Verification items for the finished model (mm, model axes). Coordinates: 2 decimals unless noted, no trailing zeros. Order: outer loops, then holes, each group sorted by start corner. A loop starts at its lowest first (then second) coordinate and runs counter-clockwise, first axis right, second up. Notation, with made-up numbers: (66, 20.5) - (89, 20.5) arc R14 ccw to (89, 37.5) - close; hole circle Ø3 at (73, 14.25). An arc over 180 degrees is marked (long way). Answer as CSV lines item,"result". Start each with the question number.
1. Section check A-A (y = 0). Record the cut outline in (x, z).
2. Section check C-C (x = 1.25). Record the cut outline in (y, z).
3. Go/stop test with flat-tipped pins: pin 1 (8 mm diameter, centred on y = -6, z = -0.5, fed in from +X); pin 2 (2 mm diameter, centred on x = 7.5, y = 5, fed in from -Z). Record where each tip stops, or that it passes through.
4. Material ranges on L1, parallel to Z at x = 7.75, y = 5.25; L2, parallel to Y at x = 7.5, z = -5.5; L3, parallel to X at y = -6.5, z = 1.5, recorded low to high. Write a range as [from, to].
5. Section check D-D (x = 3.25). Record the cut outline in (y, z), and give its area (3 significant figures).
from build123d import *

# Parameters (mm, degrees)
SKETCH_1_R       = 8
EXTRUDE_1_DEPTH  = 9
CHAMFER_1_SIZE   = 0.357142857
CHAMFER_1_SIZE_2 = 0.5
CHAMFER_2_SIZE   = 0.5


with BuildPart() as part:
    # Эскиз1 → Бобышка-Вытянуть1 (new body)
    with BuildSketch(Plane(origin=(0, 0, 0), x_dir=(0, 0, -1), z_dir=(1, 0, 0))):
        Circle(SKETCH_1_R)
    extrude(amount=EXTRUDE_1_DEPTH)

    # Эскиз2 → Вырез-Повернуть1 (revolve, cut)
    with BuildSketch(Plane.XY):
        with BuildLine():
            Line((-3, 0), (12, 0))
            ThreePointArc((12, 0), (4.5, 7.5), (-3, 0))
        make_face()
    revolve(axis=Axis((0, 0, 0), (1, 0, 0)), mode=Mode.SUBTRACT)

    # Фаска1
    # the kernel refuses this chamfer: 0.5, 0.357142857 mm, written as the material it takes off along each edge
    with BuildSketch(Plane(origin=(9, 0, 0), x_dir=(0, 1, 0), z_dir=(0, 0, 1))) as chamfer_1_piece_1:
        with BuildLine():
            Line((6 + CHAMFER_1_SIZE, 0), (6.296419414, 0.425064103))
            ThreePointArc((6.296419414, 0.425064103), (6.1560674, 0.215979206), (6, 0))
            Line((6, 0), (6 + CHAMFER_1_SIZE, 0))
        make_face()
    revolve(axis=Axis((9, 0, 0), (-1, 0, 0)), mode=Mode.SUBTRACT)
    with BuildSketch(Plane(origin=(0, 0, 0), x_dir=(0, 1, 0), z_dir=(0, 0, 1))) as chamfer_1_piece_2:
        with BuildLine():
            Line((6 + CHAMFER_1_SIZE_2, 0), (6.208166664, -0.291833336))
            ThreePointArc((6.208166664, -0.291833336), (6.10678692, -0.146018659), (6, 0))
            Line((6, 0), (6 + CHAMFER_1_SIZE_2, 0))
        make_face()
    revolve(axis=Axis((0, 0, 0), (-1, 0, 0)), mode=Mode.SUBTRACT)

    # Фаска2
    chamfer_2_edges = [part.edges().sort_by_distance(p)[0] for p in [
        (0, 0, 8),
        (9, 0, 8),
    ]]
    chamfer(chamfer_2_edges, length=CHAMFER_2_SIZE)


solid = part.part
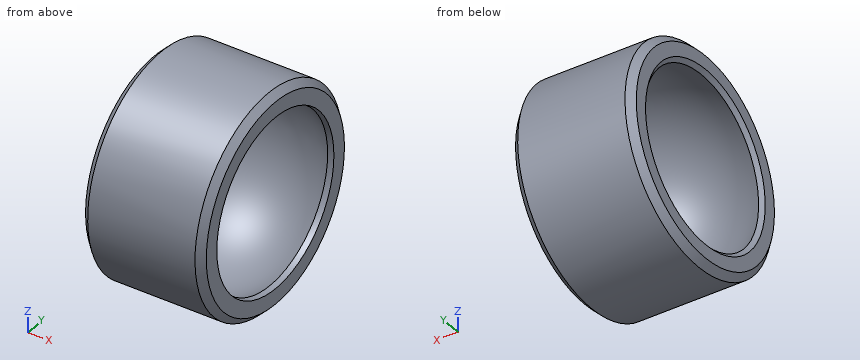
Evaluation:
1,outline,"(0, -7.5) - (0.5, -8) - (8.5, -8) - (9, -7.5) - (9, -6.36) - (8.57, -6.3) arc R7.5 cw to (0.29, -6.21) - (0, -6.5) - close; (0, 6.5) - (0.29, 6.21) arc R7.5 cw to (8.57, 6.3) - (9, 6.36) - (9, 7.5) - (8.5, 8) - (0.5, 8) - (0, 7.5) - close"
2,outline,"circle Ø16 at (0, 0); hole circle Ø13.52 at (0, 0)"
3,pin 1,"stops at x = 9"
3,pin 2,"stops at z = -6.93"
4,L1,"z = [-6.04, -4.26], [4.26, 6.04]"
4,L2,"y = [-5.81, -4.12], [4.12, 5.81]"
4,L3,"x = [0, 1.07], [7.93, 9]"
5,outline,"circle Ø16 at (0, 0); hole circle Ø14.79 at (0, 0)"
5,area,"29.3 mm²"
